Autodesk Fusion 360 part; units mm, degrees
sketch "Sketch5" plane through (0, 0, 0) normal (0, 0, 1) x (1, 0, 0)
  line L0 (25.1413, 25.1399) -> (-9.8587, 25.1399)
  line L1 (-9.8587, 25.1399) -> (-9.8587, -9.8601)
  line L2 (-9.8587, -9.8601) -> (25.1413, -9.8601)
  line L3 (25.1413, -9.8601) -> (25.1413, 25.1399)
  line L4 (-9.8587, 18.1399) -> (-24.8587, 18.1399)
  line L5 (-24.8587, 18.1399) -> (-24.8587, -1.8601)
  line L6 (-24.8587, -1.8601) -> (-9.8587, -1.8601)
  line L7 (-9.8587, -1.8601) -> (-9.8587, 18.1399)
  line L8 (25.1413, 18.1399) -> (40.1413, 18.1399)
  line L9 (40.1413, 18.1399) -> (40.1413, -1.8601)
  line L10 (40.1413, -1.8601) -> (25.1413, -1.8601)
  line L11 (25.1413, -1.8601) -> (25.1413, 18.1399)
  dimension "d12" = 35
  dimension "d13" = 35
  dimension "d14" = 15
  dimension "d15" = 20
  dimension "d16" = 7
  dimension "d17" = 15
  dimension "d18" = 20
  dimension "d19" = 7
extrude "Extrude4" add sketch "Sketch5" along normal blind 4
sketch "Sketch6" plane through (0, 0, 4) normal (0, 0, 1) x (1, 0, 0)
  line L0 (25.1413, 18.1399) -> (25.1413, 25.1399)
  line L1 (25.1413, 25.1399) -> (-9.8587, 25.1399)
  line L2 (-9.8587, 25.1399) -> (-9.8587, 18.1399)
  line L3 (-9.8587, 18.1399) -> (-24.8587, 18.1399)
  line L4 (-24.8587, 18.1399) -> (-24.8587, -1.8601)
  line L5 (-24.8587, -1.8601) -> (-9.8587, -1.8601)
  line L6 (-9.8587, -1.8601) -> (-9.8587, -9.8601)
  line L7 (-9.8587, -9.8601) -> (25.1413, -9.8601)
  line L8 (25.1413, -9.8601) -> (25.1413, -1.8601)
  line L9 (25.1413, -1.8601) -> (40.1413, -1.8601)
  line L10 (40.1413, -1.8601) -> (40.1413, 18.1399)
  line L11 (40.1413, 18.1399) -> (25.1413, 18.1399)
  circle A0 centre (-16.3587, 6.1399) radius 3
  circle A1 centre (31.6413, 6.1399) radius 3
  line L12 (7.6413, 25.1399) -> (7.6413, -9.8601) construction
  dimension "d22" = 6
  dimension "d23" = 6
  dimension "d24" = 48
  dimension "d25" = 12
  dimension "d26" = 12
  dimension "d27" = 24
extrude "Extrude5" cut sketch "Sketch6" against normal up to surface (4 mm away) contours A0 | A1
sketch "Sketch7" plane through (0, 0, 4) normal (0, 0, 1) x (1, 0, 0)
  circle A0 centre (-16.3587, 6.1399) radius 3
  circle A1 centre (31.6413, 6.1399) radius 3
  line L0 (25.1413, 18.1399) -> (25.1413, 25.1399)
  line L1 (25.1413, 25.1399) -> (-9.8587, 25.1399)
  line L2 (-9.8587, 25.1399) -> (-9.8587, 18.1399)
  line L3 (-9.8587, 18.1399) -> (-24.8587, 18.1399)
  line L4 (-24.8587, 18.1399) -> (-24.8587, -1.8601)
  line L5 (-24.8587, -1.8601) -> (-9.8587, -1.8601)
  line L6 (-9.8587, -1.8601) -> (-9.8587, -9.8601)
  line L7 (-9.8587, -9.8601) -> (25.1413, -9.8601)
  line L8 (25.1413, -9.8601) -> (25.1413, -1.8601)
  line L9 (25.1413, -1.8601) -> (40.1413, -1.8601)
  line L10 (40.1413, -1.8601) -> (40.1413, 18.1399)
  line L11 (40.1413, 18.1399) -> (25.1413, 18.1399)
  line L12 (-5.8587, 21.1399) -> (21.1413, 21.1399)
  line L13 (21.1413, 21.1399) -> (21.1413, -9.8601)
  line L14 (21.1413, -9.8601) -> (-5.8587, -9.8601)
  line L15 (-5.8587, -9.8601) -> (-5.8587, 21.1399)
  dimension "d30" = 4
  dimension "d31" = 4
  dimension "d32" = 4
sketch "Sketch9" plane through (0, 0, 4) normal (0, 0, 1) x (1, 0, 0)
  circle A0 centre (-16.3587, 6.1399) radius 3
  circle A1 centre (31.6413, 6.1399) radius 3
  line L0 (25.1413, 18.1399) -> (25.1413, 25.1399)
  line L1 (25.1413, 25.1399) -> (-9.8587, 25.1399)
  line L2 (-9.8587, 25.1399) -> (-9.8587, 18.1399)
  line L3 (-9.8587, 18.1399) -> (-24.8587, 18.1399)
  line L4 (-24.8587, 18.1399) -> (-24.8587, -1.8601)
  line L5 (-24.8587, -1.8601) -> (-9.8587, -1.8601)
  line L6 (-9.8587, -1.8601) -> (-9.8587, -9.8601)
  line L7 (-9.8587, -9.8601) -> (25.1413, -9.8601)
  line L8 (25.1413, -9.8601) -> (25.1413, -1.8601)
  line L9 (25.1413, -1.8601) -> (40.1413, -1.8601)
  line L10 (40.1413, -1.8601) -> (40.1413, 18.1399)
  line L11 (40.1413, 18.1399) -> (25.1413, 18.1399)
  line L12 (-9.8587, 25.1399) -> (25.1413, 25.1399)
  line L13 (25.1413, 25.1399) -> (25.1413, -9.8601)
  line L14 (25.1413, -9.8601) -> (-9.8587, -9.8601)
  line L15 (-9.8587, -9.8601) -> (-9.8587, 25.1399)
extrude "Extrude7" add sketch "Sketch9" along normal blind 30 contours L0 L1 L2 L6 L7 L8 L12 L13 L14 L15
extrude "Extrude6" cut sketch "Sketch7" against normal blind 4 contours L7 L12 L13 L14 L15
sketch "Sketch8" plane through (0, 0, 4) normal (0, 0, 1) x (1, 0, 0)
  line L0 (25.1413, 18.1399) -> (25.1413, -1.8601)
  line L1 (25.1413, -1.8601) -> (40.1413, -1.8601)
  line L2 (40.1413, -1.8601) -> (40.1413, 18.1399)
  line L3 (40.1413, 18.1399) -> (25.1413, 18.1399)
  line L4 (-9.8587, 18.1399) -> (-24.8587, 18.1399)
  line L5 (-24.8587, 18.1399) -> (-24.8587, -1.8601)
  line L6 (-24.8587, -1.8601) -> (-9.8587, -1.8601)
  line L7 (-9.8587, -1.8601) -> (-9.8587, 18.1399)
  circle A0 centre (-16.3587, 6.1399) radius 3
  circle A1 centre (31.6413, 6.1399) radius 3
  line L8 (-9.8587, 53.1399) -> (25.1413, 53.1399)
  line L9 (25.1413, 53.1399) -> (25.1413, 18.1399)
  line L10 (25.1413, 18.1399) -> (-9.8587, 18.1399)
  line L11 (-9.8587, 18.1399) -> (-9.8587, 53.1399)
sketch "Sketch10" plane through (0, 0, 4) normal (0, 0, -1) x (-1, 0, 0)
  line L0 (-21.1413, -9.8601) -> (5.8587, -9.8601)
  line L1 (5.8587, -9.8601) -> (5.8587, 21.1399)
  line L2 (5.8587, 21.1399) -> (-21.1413, 21.1399)
  line L3 (-21.1413, 21.1399) -> (-21.1413, -9.8601)
  line L4 (-21.1413, 21.1399) -> (5.8587, 21.1399)
  line L5 (5.8587, 21.1399) -> (5.8587, -9.8601)
  line L6 (5.8587, -9.8601) -> (-21.1413, -9.8601)
  line L7 (-21.1413, -9.8601) -> (-21.1413, 21.1399)
extrude "Extrude8" cut sketch "Sketch10" against normal up to surface (26 mm away)
fillet "Fillet1" radius 1.5 8 edges at (25.1413, 25.1399, 17) (7.6413, 25.1399, 34) (25.1413, 7.6399, 34) (-9.8587, 7.6399, 34) (-9.8587, 25.1399, 17) (25.1413, -9.8601, 17) (7.6413, -9.8601, 34) (-9.8587, -9.8601, 17)
fillet "Fillet2" radius 2 1 edges at (-9.8587, 8.1399, 4)
fillet "Fillet3" radius 2 1 edges at (-9.8587, 18.1399, 3)
fillet "Fillet4" radius 2 1 edges at (25.1413, 8.1399, 4)
fillet "Fillet5" radius 2 1 edges at (25.1413, 18.1399, 3)
fillet "Fillet6" radius 2 1 edges at (25.1413, -1.8601, 3)
fillet "Fillet7" radius 2 1 edges at (-9.8587, -1.8601, 3)
fillet "Fillet8" radius 3 1 edges at (40.1413, 18.1399, 2)
fillet "Fillet9" radius 3 1 edges at (40.1413, -1.8601, 2)
fillet "Fillet10" radius 3 1 edges at (-24.8587, 18.1399, 2)
fillet "Fillet11" radius 3.5 1 edges at (-24.8587, -1.8601, 2)
The listing builds one solid part. Answer for the finished solid, in the listing's coordinates (mm). A direction names the side the tool comes from. Give positions to 0.01 mm unless a question says otherwise; leave off trailing zeros. Order: outer loops, then holes, each group sorted by start corner. A loop starts at its lowest first (then second) coordinate and runs counter-clockwise, first axis right, second up. Notation, with made-up numbers: M 59,79.5 L 105,79.5 A15 cw 105,85.5 Z; hole C -33,63 d7. An arc over 180 degrees is marked long. Put each result on its own line as item: value. Start each with the question number.
Item 1: The part is cut by section C-C, the plane y = 10. Determine the outline of the cut face in (x, z), and give its area (3 significant figures).
Item 2: Find the intervals of material crossed by line 1 along X through (y, z) = (12.5, 16.5); line 2 along X through (y, z) = (-8, 31.5); line 3 along Y through (x, z) = (3, 19.5), in increasing order.
Item 3: The part is cut by section B-B, the plane z = 18.5. Determine the outline of the cut face in (x, y), and give its area (3 significant figures).
Item 4: Which of the six approach directions +Z, -Z, +X, -X, +Y, -Y give full straight-line access (tool end or side, diameter ignored) to faces 4 (the face through (-17, 18.14, 2)), 5 (the face through (32, 18.14, 2)), 6 (the face through (35, 8, 4))?
Item 5: Flat-ended cylindrical pins translate along their axes: P1, Ø9, axis at y = 11.5, z = 16, coming from the +X side; P2, Ø3, axis at x = -17.5, z = 2, coming from the -Y side; P3, Ø4, axis at x = -19.5, y = 9.5, coming from the +Z side. Find the tip coordinate at first contact, or state that the pin passes through.
Item 6: For a pull along X with two mould halves and no side action, classify faces 1 (the face through (7, 21.14, 15)), 2 (the face through (-17, -1.86, 2)), 3 (the face through (-10.43, 8.31, 4.6)) as +X half, -X half, draft (parallel to the pull), parting line (faces both ways), or undercut.
Item 7: The part is cut by section A-A, the plane x = 12.5. Determine the outline of the cut face in (y, z).
Item 8: The part is cut by section D-D, the plane y = 4.5. Determine the outline of the cut face in (x, z).
Answer key:
1. outline: M -24.86,0 L -5.86,0 L -5.86,30 L 21.14,30 L 21.14,0 L 40.14,0 L 40.14,4 L 27.14,4 A2 cw 25.14,6 L 25.14,32.5 A1.5 ccw 23.64,34 L -8.36,34 A1.5 ccw -9.86,32.5 L -9.86,6 A2 cw -11.86,4 L -24.86,4 Z
1. area: 501 mm²
2. line 1: x = -9.86 to -5.86, 21.14 to 25.14
2. line 2: x = -9.86 to 25.14
2. line 3: y = 21.14 to 25.14
3. outline: M -9.86,-8.36 A1.5 ccw -8.36,-9.86 L -5.86,-9.86 L -5.86,21.14 L 21.14,21.14 L 21.14,-9.86 L 23.64,-9.86 A1.5 ccw 25.14,-8.36 L 25.14,23.64 A1.5 ccw 23.64,25.14 L -8.36,25.14 A1.5 ccw -9.86,23.64 Z
3. area: 386 mm²
4. face 4: +Z, -Z, -X, +Y
4. face 5: +Z, -Z, +X, +Y
4. face 6: +Z, +X, +Y, -Y
5. P1: stops at x = 25.14
5. P2: stops at y = -1.86
5. P3: stops at z = 4
6. face 1: undercut
6. face 2: draft
6. face 3: -X half
7. outline: M -9.86,30 L 21.14,30 L 21.14,0 L 25.14,0 L 25.14,32.5 A1.5 ccw 23.64,34 L -8.36,34 A1.5 ccw -9.86,32.5 Z
8. outline: M -24.86,0 L -18.87,0 L -18.87,4 L -24.86,4 Z; M -13.85,0 L -5.86,0 L -5.86,30 L 21.14,30 L 21.14,0 L 29.13,0 L 29.13,4 L 27.14,4 A2 cw 25.14,6 L 25.14,32.5 A1.5 ccw 23.64,34 L -8.36,34 A1.5 ccw -9.86,32.5 L -9.86,6 A2 cw -11.86,4 L -13.85,4 Z; M 34.15,0 L 40.14,0 L 40.14,4 L 34.15,4 Z
